Source: CAD feature listing. Evaluate the final solid. Frame: model axes, mm. A direction names the side the tool comes from. Round coordinates to 2 decimals unless told otherwise and drop trailing zeros. Order: outer loops, then holes, each group sorted by start corner. A loop starts at its lowest first (then second) coordinate and runs counter-clockwise, first axis right, second up. Notation, with made-up numbers: (48.5, 50.25) - (78.5, 50.25) arc R25 ccw to (78.5, 76.25) - close; hole circle Ø8 at (-23, 78.25). An arc over 180 degrees is marked (long way). Put each result on its own line as item: value. Start each with the question number.
1) Section C-C on y = -9.5. Output: boundary loops of the cut face in (x, z) (1 decimal), then the cut area to 3 significant figures.
2) Mould query, pull axis Z, two halves, no side actions, for faces 1 (the face through (70, 5.193, 63)), 2 (the face through (75.587, 2.778, 57.958)), 3 (the face through (-67.799, -29, 0)). Classes: +Z half, -Z half, draft (parallel to the pull), parting line (faces both ways), or undercut.
3) Line query: probe 1 along X at (y, z) = (-28, 0); probe 2 along X at (y, z) = (4.5, 0). Output: solid intervals per line, ascending. Write a range as [from, to].
4) Section A-A on x = 0. Output: boundary loops of the cut face in (y, z), then the cut area to 3 significant figures.
5) Section B-B on z = -12. Output: boundary loops of the cut face in (x, y), then the cut area to 3 significant figures.
6) Contact query for flat-ended pins moving along their axis: P1, Ø8, axis at y = -4.5, z = -32.5, coming from the -X side; P2, Ø4, axis at y = -25.5, z = 59, coming from the +X side; P3, Ø2.5, axis at y = -29.5, z = -2, coming from the -X side. Output: stop coordinate, or through.
7) Section D-D on z = -54. Output: boundary loops of the cut face in (x, y).
8) Access query for faces 4 (the face through (-89.34, -15.67, -28.13)), 5 (the face through (-77, -29, -25.4)), 6 (the face through (1, -31.319, 20)), 7 (the face through (-90.434, -13.613, -3.11)). Directions: +Z, -Z, +X, -X, +Y, -Y. A direction counts if a zero-diameter tool reaches every point of the face in a straight line with its end or side. Return the directions, or none.
```python
from build123d import *

# Parameters (mm, degrees)
CUT_EXTRUDE1_DEPTH = 25.4


with BuildPart() as part:
    # Sketch1 → Revolve1 (revolve)
    with BuildSketch(Plane.XY):
        Polygon((-95.25, 5.193008475), (-95.25, 0.430508475), (-93.6625, 0.430508475), (-93.6625, -31.319491525), (0, -31.319491525), (0, -26.556991525), (-90.4875, -26.556991525), (-90.4875, 3.605508475), (-93.6625, 3.605508475), (-93.6625, 5.193008475), align=None)
    revolve(axis=Axis((0, 0, 0), (0, -1, 0)))

    # Sketch7 → 5/8 (0.625) Diameter Hole1 (revolve, cut)
    with BuildSketch(Plane(origin=(0, -26.556991525, 0), x_dir=(0, 0, 1), z_dir=(1, 0, 0))):
        Polygon((0, 0), (0, 4.7625), (7.9375, 4.7625), (7.9375, 0.532828266), (8.5725, 0), align=None)
    revolve(axis=Axis((0, -20.206991525, 0), (0, -1, 0)), mode=Mode.SUBTRACT)

    # Sketch12 → Cut-Extrude1 (cut)
    with BuildSketch(Plane(origin=(0, -26.556991525, 0), x_dir=(1, 0, 0), z_dir=(0, 1, 0))):
        with BuildLine():
            Line((-86.849453978, 25.4), (-67.799453978, 25.4))
            Line((-67.799453978, 25.4), (-67.799453978, -25.4))
            Line((-67.799453978, -25.4), (-86.849453978, -25.4))
            ThreePointArc((-86.849453978, -25.4), (-90.4875, 0), (-86.849453978, 25.4))
        make_face()
    extrude(amount=-CUT_EXTRUDE1_DEPTH, mode=Mode.SUBTRACT)


solid = part.part
```
Answer sheet:
1. outline: circle Ø187.3 at (0, 0); hole circle Ø181 at (0, 0)
1. area: 1,840 mm^2
2. face 1: draft
2. face 2: parting line
2. face 3: undercut
3. probe 1: [-93.66, -90.49], [-67.8, -7.94], [7.94, 93.66]
3. probe 2: [-95.25, -93.66], [93.66, 95.25]
4. outline: (-31.32, -93.66) - (0.43, -93.66) - (0.43, -95.25) - (5.19, -95.25) - (5.19, -93.66) - (3.61, -93.66) - (3.61, -90.49) - (-26.56, -90.49) - (-26.56, -8.57) - (-27.09, -7.94) - (-31.32, -7.94) - close; (-31.32, 7.94) - (-27.09, 7.94) - (-26.56, 8.57) - (-26.56, 90.49) - (3.61, 90.49) - (3.61, 93.66) - (5.19, 93.66) - (5.19, 95.25) - (0.43, 95.25) - (0.43, 93.66) - (-31.32, 93.66) - close
4. area: 1,020 mm^2
5. outline: (-94.49, 0.43) - (-92.89, 0.43) - (-92.89, -31.32) - (-89.69, -31.32) - (-89.69, 3.61) - (-92.89, 3.61) - (-92.89, 5.19) - (-94.49, 5.19) - close; (-67.8, -31.32) - (92.89, -31.32) - (92.89, 0.43) - (94.49, 0.43) - (94.49, 5.19) - (92.89, 5.19) - (92.89, 3.61) - (89.69, 3.61) - (89.69, -26.56) - (-67.8, -26.56) - close
5. area: 989 mm^2
6. P1: x = -89.22
6. P2: x = 74.32
6. P3: x = -93.66
7. outline: (-78.46, 0.43) - (-76.53, 0.43) - (-76.53, -31.32) - (76.53, -31.32) - (76.53, 0.43) - (78.46, 0.43) - (78.46, 5.19) - (76.53, 5.19) - (76.53, 3.61) - (72.61, 3.61) - (72.61, -26.56) - (-72.61, -26.56) - (-72.61, 3.61) - (-76.53, 3.61) - (-76.53, 5.19) - (-78.46, 5.19) - close
8. face 4: -Y
8. face 5: +Y, -Y
8. face 6: +Z, -Z, +X, -X, -Y
8. face 7: +Y
